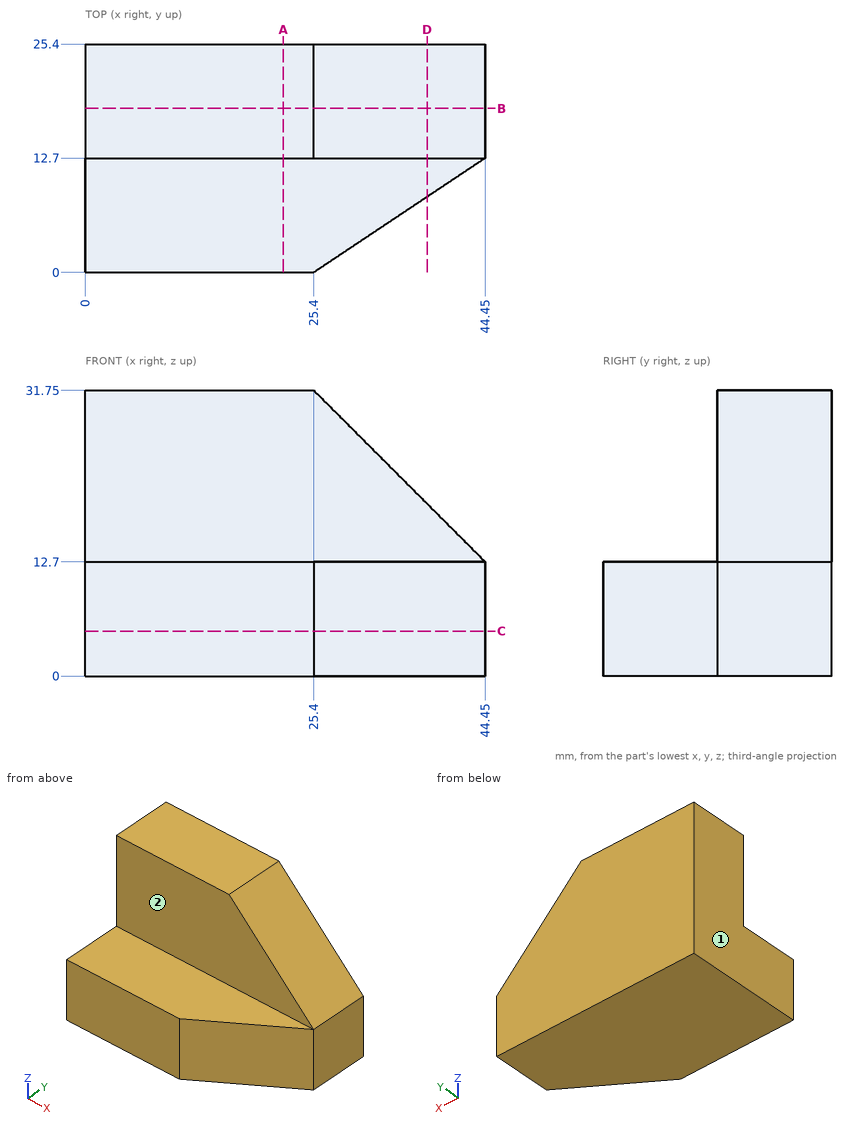
Geometry: see drawing. Coordinates: mm, zero at the bounding-box minimum. A direction names the side the tool comes from. Coordinates: 2 decimals unless noted, no trailing zeros. Loops run counter-clockwise (first coordinate to the right, second up) from the corner with the lowest first, then second, coordinate; pieces in that order, holes last. Notation, with made-up numbers: (1, -21) - (24, -21) arc R30 cw to (24, 11) - close; hole circle Ø10 at (32, 1). An arc over 180 degrees is marked (long way). Return JSON: item names as keys, results as strings.
Q1. Section D-D, the plane x = 38. Return loops of the section in (y, z).
Results:
{"outline": "(8.4, 0) - (25.4, 0) - (25.4, 19.15) - (12.7, 19.15) - (12.7, 12.7) - (8.4, 12.7) - close"}
Q2. Contact query for flat-ended pins moving along their axis: P1, Ø2, axis at x = 15, y = 9, coming from the -Z side; P2, Ø10, axis at x = 27, y = 5.5, coming from the +Z side; P3, Ø3, axis at x = 33.5, y = 21.5, coming from the +Z side; P4, Ø6, axis at x = 39, y = 3, coming from the +Z side. Output: stop coordinate, or through.
Results:
{"P1": "z = 0", "P2": "z = 12.7", "P3": "z = 25.15", "P4": "through"}
Q3. Section C-C, the plane z = 5. Return loops of the section in (x, y).
Results:
{"outline": "(0, 0) - (25.4, 0) - (44.45, 12.7) - (44.45, 25.4) - (0, 25.4) - close"}
Q4. Section B-B, the plane y = 18.25. Return loops of the section in (x, z), plus the area to 3 significant figures.
Results:
{"outline": "(0, 0) - (44.45, 0) - (44.45, 12.7) - (25.4, 31.75) - (0, 31.75) - close", "area": "1,230 mm2"}
Q5. Material intervals for line 1 along Z through (x, y) = (8, 5.25); line 2 along Y through (x, z) = (26, 22.5); line 3 along Z through (x, y) = (37.5, 22.5), sorted ascending.
Results:
{"line 1": "0 to 12.7", "line 2": "12.7 to 25.4", "line 3": "0 to 19.65"}
Q6. Section A-A, the plane x = 22. Return loops of the section in (y, z), plus the area to 3 significant figures.
Results:
{"outline": "(0, 0) - (25.4, 0) - (25.4, 31.75) - (12.7, 31.75) - (12.7, 12.7) - (0, 12.7) - close", "area": "565 mm2"}
Q7. Access query for the marked faces 1 and 2. Directions: +Z, -Z, +X, -X, +Y, -Y. A direction counts if a zero-diameter tool reaches every point of the face in a straight line with its end or side. Return the directions, or none.
Results:
{"face 1": "+Z, -Z, -X, +Y, -Y", "face 2": "+Z, +X, -X, -Y"}
